```python
from build123d import *

# Parameters (mm, degrees)
SKETCH2_W           = 107
SKETCH2_H           = 107
BOSS_EXTRUDE1_DEPTH = 8
SKETCH14_W          = 107
SKETCH14_H          = 107
BOSS_EXTRUDE2_DEPTH = 18
SKETCH15_W          = 102.5
SKETCH15_H          = 102.5
CUT_EXTRUDE4_DEPTH  = 20
SKETCH12_W          = 20.6
SKETCH12_H          = 90.000135975
CUT_EXTRUDE3_DEPTH  = 4.1


with BuildPart() as part:
    # Sketch2 → Boss-Extrude1 (new body)
    with BuildSketch(Plane(origin=(0, 0, 0), x_dir=(1, 0, 0), z_dir=(0, 1, 0))):
        Rectangle(SKETCH2_W, SKETCH2_H)
    extrude(amount=BOSS_EXTRUDE1_DEPTH)

    # Sketch14 → Boss-Extrude2 (add)
    with BuildSketch(Plane(origin=(0, 8, 0), x_dir=(1, 0, 0), z_dir=(0, 1, 0))):
        Rectangle(SKETCH14_W, SKETCH14_H)
    extrude(amount=BOSS_EXTRUDE2_DEPTH)

    # Sketch15 → Cut-Extrude4 (cut)
    with BuildSketch(Plane(origin=(0, 26, 0), x_dir=(1, 0, 0), z_dir=(0, 1, 0))):
        Rectangle(SKETCH15_W, SKETCH15_H)
    extrude(amount=-CUT_EXTRUDE4_DEPTH, mode=Mode.SUBTRACT)

    # Sketch12 → Cut-Extrude3 (cut)
    with BuildSketch(Plane(origin=(0, 6, 0), x_dir=(1, 0, 0), z_dir=(0, 1, 0))):
        with Locations((0, -8.499932013)):
            Rectangle(SKETCH12_W, SKETCH12_H)
    extrude(amount=-CUT_EXTRUDE3_DEPTH, mode=Mode.SUBTRACT)


solid = part.part
```
Can you work these out from the model? Positions are in its coordinate system, mm. A direction names the side the tool comes from. Give positions to 0.01 mm unless a question says otherwise; leave off trailing zeros. Order: outer loops, then holes, each group sorted by start corner. A loop starts at its lowest first (then second) coordinate and runs counter-clockwise, first axis right, second up. Notation, with made-up numbers: M 48.25,7 L 85.25,7 A9 cw 85.25,15 Z; hole C 49,81.5 d3. An arc over 180 degrees is marked long. Write item = value, one per line. Start each with the question number.
Q1. Suppose I cut it at B-B (z = 6). Write out the boundary of the cut face in (x, y), plus the area to 3 significant figures.
Q2. Suppose I cut it at D-D (y = 4.5). Write out the boundary of the cut face in (x, z).
Q3. We'd pull the mould along X, two halves only. Please class faces 4 (the flat face through (53.5, 13, 1)), 5 (the flat face through (-10.3, 4, 9)), 6 (the flat face through (-1, 13, -53.5)): pulls with the +X half, pulls with the -X half, needs draft (parallel to the pull), parting line crosses it, or undercut.
Q4. I need wall thicknesses on probe 1 along X at (y, z) = (5, 1.5); probe 2 along X at (y, z) = (15.5, 40). Which ranges of each line are inside material? Lowest first, please. Write a range as [from, to].
Q5. Suppose I cut it at C-C (y = 22.25). Write out the boundary of the cut face in (x, z).
Q6. Will these pins go through, and if not, where does the flat tip stop? pin 1 Ø22.5 at (x, z) = (3.5, 27) entering from +Y; pin 2 Ø8 at (x, z) = (2.5, 17) entering from +Y; pin 3 Ø3.5 at (x, y) = (-3, 3.5) entering from +Z.
Q7. For faces 1 (the flat face through (-1, 16, 51.25)), 2 (the flat face through (-53.5, 13, 1)), 3 (the flat face through (0, 4, -36.5)), which set-ups out of +Z, -Z, +X, -X, +Y, -Y let a thin tool reach every point of the face, with its end or its side?
Q8. Suppose I cut it at A-A (x = -2). Write out the boundary of the cut face in (y, z).
Check result:
q1.outline = M -53.5,0 L 53.5,0 L 53.5,26 L 51.25,26 L 51.25,6 L 10.3,6 L 10.3,1.9 L -10.3,1.9 L -10.3,6 L -51.25,6 L -51.25,26 L -53.5,26 Z
q1.area = 648 mm2
q2.outline = M -53.5,-53.5 L 53.5,-53.5 L 53.5,53.5 L 10.3,53.5 L 10.3,-36.5 L -10.3,-36.5 L -10.3,53.5 L -53.5,53.5 Z
q3.face_4 = pulls with the +X half
q3.face_5 = undercut
q3.face_6 = needs draft
q4.probe_1 = [-53.5, -10.3], [10.3, 53.5]
q4.probe_2 = [-53.5, -51.25], [51.25, 53.5]
q5.outline = M -53.5,-53.5 L 53.5,-53.5 L 53.5,53.5 L -53.5,53.5 Z; hole M -51.25,-51.25 L 51.25,-51.25 L 51.25,51.25 L -51.25,51.25 Z
q6.pin_1 = 6
q6.pin_2 = 1.9
q6.pin_3 = 53.5
q7.face_1 = +Y
q7.face_2 = +Z, -Z, -X, +Y, -Y
q7.face_3 = +Z, +Y
q8.outline = M 0,-53.5 L 26,-53.5 L 26,-51.25 L 6,-51.25 L 6,-36.5 L 1.9,-36.5 L 1.9,53.5 L 0,53.5 Z; M 6,51.25 L 26,51.25 L 26,53.5 L 6,53.5 Z
